from build123d import *

# Parameters (mm, degrees)
EXTRUDE_1_DEPTH              = 50
HOLE_WIZARD_M4_1_D           = 4.5
HOLE_WIZARD_M4_1_CBORE_D     = 7.7
HOLE_WIZARD_M4_1_CBORE_DEPTH = 2.9


with BuildPart() as part:
    # ｽｹｯﾁ1 → ﾎﾞｽ - 押し出し1 (new body)
    with BuildSketch(Plane.XY):
        Polygon((0, 0), (4.4, 0), (6.520098337, 2.120098337), (10.279901663, 2.120098337), (12.4, 0), (16.8, 0), (16.8, 2.6), (14, 2.6), (14, 5.2), (2.8, 5.2), (2.8, 2.6), (0, 2.6), align=None)
    extrude(amount=EXTRUDE_1_DEPTH)

    # M4 丸平ねじ用座ぐり穴1 (through all)
    with Locations(Plane(origin=(8.4, 5.2, 10), x_dir=(1, 0, 0), z_dir=(0, 1, 0))):
        with Locations((0, 0), (0, -30)):
            CounterBoreHole(HOLE_WIZARD_M4_1_D / 2, HOLE_WIZARD_M4_1_CBORE_D / 2, HOLE_WIZARD_M4_1_CBORE_DEPTH)


solid = part.part
Source: CAD feature listing. Evaluate the final solid. Frame: model axes, mm. A direction names the side the tool comes from. Coordinates: 2 decimals unless noted, no trailing zeros. Order: outer loops, then holes, each group sorted by start corner. A loop starts at its lowest first (then second) coordinate and runs counter-clockwise, first axis right, second up. Notation, with made-up numbers: M 27.5,28.25 L 36.5,28.25 A12 ccw 36.5,49.25 Z; hole C -29,40 d6. An arc over 180 degrees is marked long. Write each question's results on one line, items separated by ' | '. Start each with the question number.
Item 1: Draft query along Z for faces 4 (the face through (10, 2.3, 42)), 5 (the face through (2.8, 4, 25)), 6 (the face through (8, 3, 0)), 7 (the face through (10.177, 3.77, 43.416)). Return one class per face: pulls with the +Z half, pulls with the -Z half, needs draft (parallel to the pull), parting line crosses it, or undercut.
Item 2: Line query: probe 1 along X at (y, z) = (2.05, 10); probe 2 along X at (y, z) = (4.1, 40); probe 3 along Z at (x, y) = (7.75, 3.5). Output: solid intervals per line, ascending.
Item 3: Cut plane C-C (y = 3.05). Return loops of the section in (x, z), and give its area (3 significant figures).
Item 4: Cut plane D-D (z = 30.5). Return loops of the section in (x, y).
Item 5: First-contact query: pin 1 Ø3 at (y, z) = (3.5, 34) entering from +X; pin 2 Ø7 at (x, z) = (8.4, 10) entering from +Y; pin 3 Ø1.1 at (x, z) = (9.5, 19.5) entering from -Y; pin 4 Ø6 at (x, z) = (8.4, 40) entering from -Y. Flat tips, straight axial feed; report the tip coordinate or a pass-through.
Item 6: Set-up query: faces 1 (the face through (8, 2.12, 46)), 2 (the face through (10, 2.3, 12)), 3 (the face through (14, 4, 25)). Return all of +Z, -Z, +X, -X, +Y, -Y with unobstructed straight access to the full face (end or side cutting, diameter ignored); none if empty.
Item 7: Cut plane B-B (z = 40). Return loops of the section in (x, y), and give its area (3 significant figures).
Item 8: Cut plane A-A (x = 8.4). Return loops of the section in (y, z).
Checked values:
1) face 4: undercut | face 5: needs draft | face 6: pulls with the -Z half | face 7: undercut
2) probe 1: x = 0 to 6.15, 10.65 to 16.8 | probe 2: x = 2.8 to 4.55, 12.25 to 14 | probe 3: z = 0 to 6.21, 13.79 to 36.21, 43.79 to 50
3) outline: M 2.8,0 L 14,0 L 14,50 L 2.8,50 Z; hole C 8.4,10 d7.7; hole C 8.4,40 d7.7 | area: 467 mm2
4) outline: M 0,0 L 4.4,0 L 6.52,2.12 L 10.28,2.12 L 12.4,0 L 16.8,0 L 16.8,2.6 L 14,2.6 L 14,5.2 L 2.8,5.2 L 2.8,2.6 L 0,2.6 Z
5) pin 1: stops at x = 16.8 | pin 2: stops at y = 2.3 | pin 3: stops at y = 2.12 | pin 4: stops at y = 1
6) face 1: +Z, -Z, -Y | face 2: +Y | face 3: +Z, -Z, +X, +Y
7) outline: M 0,0 L 4.4,0 L 6.15,1.75 L 6.15,2.3 L 4.55,2.3 L 4.55,5.2 L 2.8,5.2 L 2.8,2.6 L 0,2.6 Z; M 10.65,1.75 L 12.4,0 L 16.8,0 L 16.8,2.6 L 14,2.6 L 14,5.2 L 12.25,5.2 L 12.25,2.3 L 10.65,2.3 Z | area: 37.1 mm2
8) outline: M 2.12,0 L 5.2,0 L 5.2,6.15 L 2.3,6.15 L 2.3,7.75 L 2.12,7.75 Z; M 2.12,12.25 L 2.3,12.25 L 2.3,13.85 L 5.2,13.85 L 5.2,36.15 L 2.3,36.15 L 2.3,37.75 L 2.12,37.75 Z; M 2.12,42.25 L 2.3,42.25 L 2.3,43.85 L 5.2,43.85 L 5.2,50 L 2.12,50 Z
